Autodesk Inventor part; units mm, degrees
ref_plane "Work Plane1" through (30.1625, 0, 0) normal (0, 0, -1) x (1, 0, 0)
ref_plane "YZ Plane" through (0, 0, 0) normal (1, 0, 0) x (0, 1, 0)
ref_plane "XZ Plane" through (0, 0, 0) normal (0, 1, 0) x (-1, 0, 0)
sketch "Эскиз1" plane through (0, 0, 0) normal (0, 0, 1) x (1, 0, 0)
  line L0 (-6, 0) -> (20, 0)
  line L1 (20, 0) -> (20, 5)
  line L2 (20, 5) -> (1.5, 5)
  line L3 (1.5, 5) -> (0.5798, 5)
  line L4 (0.5798, 5) -> (0, 5)
  line L5 (0, 5) -> (0, 8)
  line L6 (-11.2, 0) -> (25.2, 0)
  line L7 (0, -1.6) -> (0, 9.6)
  line L8 (-6, 0) -> (-6, 8)
  line L9 (0, 8) -> (-6, 8)
  dimension "d0" = 20
  dimension "d1" = 18.5
  dimension "d2" = 0.9202
  dimension "d3" = 6
  dimension "d4" = 10
  dimension "d5" = 10
  dimension "d9" = 16
  dimension "d10" = 0
revolve "Базовый элемент" add sketch "Эскиз1" angle 360 about axis through (-6, 0, 0) along (1, 0, 0)
sketch "Эскиз2" plane through (-6, 0, 0) normal (-1, 0, 0) x (0, 0, 1)
  circle A0 centre (0, 0) radius 8
  line L0 (0, 0) -> (0, 8)
  line L1 (-8, 1.05) -> (8, 1.05)
  line L2 (8, 1.05) -> (8, -1.05)
  line L3 (8, -1.05) -> (-8, -1.05)
  line L4 (-8, -1.05) -> (-8, 1.05)
  line L5 (-8, 0) -> (8, 0) construction
  line L6 (0, 1.05) -> (0, -1.05) construction
  dimension "d11" = 2.1
  dimension "d12" = 16
fillet "Сопряжение1" radius 0.01 1 edges at (-6, -8, 0)
extrude "Паз" cut sketch "Эскиз2" against normal blind 4.2 contours A0 L3 L1 | L2 L3 A0 | A0 L1 L2 | L3 L4 A0 | A0 L4 L1
thread "Резьба"
chamfer "Chamfer4" distance 1 angle 45 1 edges at (20, -5, 0)
ref_plane "Work Plane1" through (30.1625, 0, 0) normal (0, 0, -1) x (1, 0, 0)
equation "\"d11\" = SBR"
equation "\"d12\" = KOD"
equation "\"d13\" = RR"
equation "\"d16\" = STI"
equation "\"d14\" = GEL"
equation "\"d40\" = 0.1 * GD"
equation "\"d0\" = NLG"
equation "\"d1\" = GEL"
equation "\"d2\" = GAL"
equation "\"d3\" = KOH"
equation "\"d4\" = GD"
equation "\"d5\" = BDM"
equation "\"d9\" = KOD"
equation "\"GD\" = NND"
equation "\"NLG\" = 20"
equation "\"GEL\" = 18.5"
equation "\"KOD\" = 16"
equation "\"KOH\" = 6"
equation "\"GAL\" = 0.61345 * PTC"
equation "\"BDM\" = NND"
equation "\"RR\" = 0.01"
equation "\"SBR\" = 2.1"
equation "\"STI\" = 4.2"
equation "\"KEWI\" = 0"
equation "\"GUL\" = 0.61345 * PTC"
equation "\"SPD\" = NND - 1.2269 * PTC"
equation "\"PTC\" = 1.5"
equation "\"TOA\" = 30deg"
equation "\"FAWI\" = 45deg"
equation "\"GD1\" = THREADDIA - 1.2269 * PTC"
properties part number "Винт M10-6gx20 ГОСТ 1491-80" material "Сталь, мягкая"
Geometry: final body of the model. Coordinates: model frame, mm. A direction names the side the tool comes from. Round coordinates to 2 decimals unless told otherwise and drop trailing zeros. Write each loop counter-clockwise with the first axis right and the second up, starting at its lowest first coordinate (ties: lowest second). Pieces come first, ordered by that corner, then holes. Notation, with made-up numbers: (-11.5, 81.25) -> (-5.5, 81.25) arc R20 ccw to (-5.5, 97.25) -> close; hole circle Ø6 at (56, 83). An arc over 180 degrees is marked (long way). Return JSON: item names as keys, results as strings.
Q1. First-contact query: pin 1 Ø1.3 at (x, z) = (-4.5, 1) entering from -Y; pin 2 Ø8 at (x, y) = (15, 4) entering from +Z; pin 3 Ø4 at (x, z) = (11.5, -1.5) entering from +Y. Flat tips, straight axial feed; report the tip coordinate or a pass-through.
From the geometry:
{"pin 1": "y = -7.99", "pin 2": "z = 5", "pin 3": "y = 5"}
Q2. Mould query, pull axis Y, two halves, no side actions, for faces 4 (the flat face through (-1.8, 0, 0)), 5 (the flat face through (-6, 4, 0)), 6 (the cylindrical face through (9.37, -1.08, 4.88)). Classes: +Y half, -Y half, draft (parallel to the pull), parting line (faces both ways), or undercut.
From the geometry:
{"face 4": "undercut", "face 5": "draft", "face 6": "parting line"}
Q3. Section D-D on x = 12. Return the cut outline in (y, z), and give its area (3 significant figures).
From the geometry:
{"outline": "circle Ø10 at (0, 0)", "area": "78.5 mm2"}
Q4. Ray query, line 1 (X direction, y = 0, z = 2.5); line 2 (Y direction, x = -1.75, z = -1); line 3 (X direction, y = 6.25, z = 4.5). Return the intervals inside material, ascending.
From the geometry:
{"line 1": "-1.8 to 20", "line 2": "-7.94 to 7.94", "line 3": "-6 to 0"}
Q5. Set-up query: faces 1 (the cylindrical face through (-3.04, -1.73, 7.81)), 2 (the flat face through (-4, 1.05, 0)), 3 (the flat face through (0, -0.1, -5.2)). Return all of +Z, -Z, +X, -X, +Y, -Y with unobstructed straight access to the full face (end or side cutting, diameter ignored); none if empty.
From the geometry:
{"face 1": "+X, -X", "face 2": "+Z, -Z, -X", "face 3": "+X"}
Q6. Section C-C on x = -0.5. Return the cut outline in (y, z), and give its area (3 significant figures).
From the geometry:
{"outline": "circle Ø16 at (0, 0)", "area": "201 mm2"}
Q7. Section A-A on y = 0. Return the cut outline in (x, z), and give its area (3 significant figures).
From the geometry:
{"outline": "(-1.8, -8) -> (0, -8) -> (0, -5) -> (19, -5) -> (20, -4) -> (20, 4) -> (19, 5) -> (0, 5) -> (0, 8) -> (-1.8, 8) -> close", "area": "228 mm2"}
